CAD build for the part. Positions are in the model's coordinates, mm. Give positions to 0.01 mm unless a question says otherwise; leave off trailing zeros. Loops run counter-clockwise (first coordinate to the right, second up) from the corner with the lowest first, then second, coordinate; pieces in that order, holes last. Notation, with made-up numbers: (50, -3.5) - (83, -3.5) arc R27 cw to (83, 13.5) - close; hole circle Ø10 at (-39.5, 56). An arc over 180 degrees is marked (long way). Return JSON: item names as keys, results as strings.
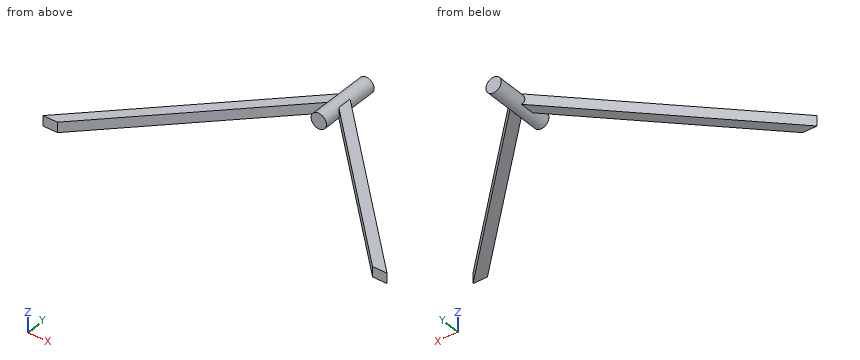
from build123d import *

# Parameters (mm, degrees)
SKETCH2_R           = 19.05
BOSS_EXTRUDE1_DEPTH = 152.4
BOSS_EXTRUDE2_DEPTH = 12.7


with BuildPart() as part:
    # Sketch2 → Boss-Extrude1 (new body)
    with BuildSketch(Plane(origin=(0, 0, 0), x_dir=(1, 0, 0), z_dir=(0, 1, 0))):
        with Locations(Location((0, 0, 0), (0, 0, 90))):
            Circle(SKETCH2_R)
    extrude(amount=BOSS_EXTRUDE1_DEPTH)

    # Sketch3 → Boss-Extrude2 (add, symmetric)
    with BuildSketch(Plane.XY):
        Polygon((-427.750314484, -331.6732), (-409.789802242, -313.712687758), (-391.82929, -331.6732), align=None)
        Polygon((-6.028675512, 90.048438972), (-409.789802242, -313.712687758), (-391.82929, -331.6732), (11.93183673, 72.08792673), align=None)
    boss_extrude2 = extrude(amount=BOSS_EXTRUDE2_DEPTH, both=True)

    # Mirror1: Boss-Extrude2 across plane
    add(boss_extrude2.mirror(Plane(origin=(0, 0, 0), x_dir=(0, 0, 1), z_dir=(1, 0, 0))))


solid = part.part
1. Drop flat-ended pins along their axis: P1, Ø6, axis at y = 51.5, z = 7, coming from the +X side; P2, Ø1, axis at x = -314.5, z = 6, coming from the -Y side; P3, Ø8, axis at x = -275, z = 6, coming from the -Y side. Give the stop position or say it passes through.
Values follow:
{"P1": "stops at x = 47.58", "P2": "stops at y = -254.84", "P3": "stops at y = -218.84"}
2. Cut at D-D, the plane x = -222.5. Write the cut outline in (y, z), plus the area to 3 significant figures.
Values follow:
{"outline": "(-162.34, -12.7) - (-126.42, -12.7) - (-126.42, 12.7) - (-162.34, 12.7) - close", "area": "912 mm²"}
3. Cut at C-C, the plane x = 0. Write the cut outline in (y, z).
Values follow:
{"outline": "(0, -19.05) - (152.4, -19.05) - (152.4, 19.05) - (0, 19.05) - close"}
4. Cut at A-A, the plane y = -186.5. Write the cut outline in (x, z).
Values follow:
{"outline": "(-282.58, -12.7) - (-246.66, -12.7) - (-246.66, 12.7) - (-282.58, 12.7) - close; (246.66, -12.7) - (282.58, -12.7) - (282.58, 12.7) - (246.66, 12.7) - close"}
5. Cut at B-B, the plane z = -1. Write the cut outline in (x, y).
Values follow:
{"outline": "(-427.75, -331.67) - (-391.83, -331.67) - (-19.02, 41.13) - (-19.02, 0) - (19.02, 0) - (19.02, 41.13) - (391.83, -331.67) - (427.75, -331.67) - (19.02, 77.05) - (19.02, 152.4) - (-19.02, 152.4) - (-19.02, 77.05) - close"}
6. Drill centre lines: probe 1 along Z at (x, y) = (95, -21); probe 2 along Y at (x, z) = (7.5, 17); probe 3 along X at (y, z) = (-125, 3). Where is each one in solid material? Low to high.
Values follow:
{"probe 1": "z = -12.7 to 12.7", "probe 2": "y = 0 to 152.4", "probe 3": "x = -221.08 to -185.16, 185.16 to 221.08"}
